For this review, take the finished solid that the model builds, in its own axes (mm). Round coordinates to 2 decimals unless told otherwise and drop trailing zeros. Loops run counter-clockwise (first coordinate to the right, second up) from the corner with the lowest first, then second, coordinate; pieces in that order, holes last.
1. Consider section C-C on x = 186. State the section outline as (y, z) points.
2. To check wall thickness, follow line 1 along Y through (x, z) = (236, -27); line 2 along Y through (x, z) = (59.5, -41); line 3 along Z through (x, y) = (119.5, -5). State the ranges of each line that lie inside material, in increasing order.
3. Clearance check with flat-ended pins moving along their axes: pin 1 Ø10 at (x, z) = (93.5, -4) entering from +Y; pin 2 Ø1.5 at (x, z) = (66.5, -39.5) entering from -Y; pin 3 Ø8 at (x, y) = (265, -23.5) entering from -Z. State where each tip first meets the part, or that it passes through.
4. Consider section B-B on z = -31. State the section outline as (x, y) points, then the cut area to 3 significant figures.
Autodesk Inventor part; units mm, degrees
ref_plane "YZ Plane" through (0, 0, 0) normal (1, 0, 0) x (0, 1, 0)
ref_plane "XZ Plane" through (0, 0, 0) normal (0, 1, 0) x (-1, 0, 0)
ref_plane "XY Plane" through (0, 0, 0) normal (0, 0, 1) x (1, 0, 0)
sketch "草圖3" plane through (0, 0, 0) normal (0, 1, 0) x (-1, 0, 0)
  line L0 (0, 50) -> (-450, 50)
  line L1 (-450, 50) -> (-450, -50)
  line L2 (-450, -50) -> (0, -50)
  line L3 (0, -50) -> (0, 50)
  point P0 (0, 0)
  point P1 (0, 0)
  dimension "d17" = 100
  dimension "d18" = 450
extrude "擠出3" add sketch "草圖3" along normal mid plane 100
chamfer "倒角4" distance 50 distance2 70 1 edges at (0, 0, 50) measured on face at (0, -16.6667, -16.6667)
chamfer "倒角5" distance 70 distance2 50 1 edges at (0, -50, -25) measured on face at (173.3333, -50, -16.6667)
chamfer "倒角6" distance 70 distance2 50 1 edges at (0, 25, -50) measured on face at (173.3333, 16.6667, -50)
chamfer "倒角8" distance 50 distance2 380 1 edges at (450, 0, -50) measured on face at (450, 16.6667, -16.6667)
chamfer "倒角9" distance 380 distance2 50 1 edges at (450, 50, 25) measured on face at (196.6667, 50, 0)
chamfer "倒角10" distance 50 distance2 380 1 edges at (450, -25, 50) measured on face at (450, -33.3333, 33.3333)
sketch "草圖4" plane through (0, 0, 0) normal (0, 0, 1) x (1, 0, 0)
  line L0 (450, -50) -> (70, -50)
  line L1 (450, 0) -> (70, 50)
  line L2 (70, -50) -> (450, 0)
  line L3 (450, 0) -> (450, -50)
  line L4 (450, 0) -> (450, -50)
  line L5 (450, -50) -> (70, -50)
  point P0 (0, 0)
  point P1 (70, 50)
  point P2 (170, -50)
  point P3 (170, 50)
extrude "擠出4" cut sketch "草圖4" along normal mid plane 100
sketch "草圖5" plane through (0, 0, 0) normal (0, 0, 1) x (1, 0, 0)
  line L0 (70, -50) -> (0, 0)
  line L1 (0, 50) -> (0, 0)
  line L2 (0, 0) -> (0, 50)
  line L3 (70, 50) -> (70, -50)
  line L4 (0, 50) -> (70, 50)
  line L5 (70, 50) -> (0, 0)
extrude "擠出5" cut sketch "草圖5" along normal mid plane 100 contours L1 L4 L5
sketch "草圖6" plane through (0, 0, 0) normal (1, 0, 0) x (0, 1, 0)
  circle A0 centre (0, 0) radius 25
  line L0 (0, 25) -> (0, -25)
  point P0 (0, 0)
  dimension "d46" = 50
revolve "迴轉1" add sketch "草圖6" angle 360 about axis through (0, 0, 25) along (0, 0, -1) picked at (-8.8525, -4.4917) contours L0 A0
sketch "草圖7" plane through (0, 0, 0) normal (0, 1, 0) x (-1, 0, 0)
  line L0 (-450, 0) -> (-70, -50)
  circle A0 centre (-450, 0) radius 15
  line L1 (-450, 15) -> (-450, -15)
  point P0 (0, 0)
  dimension "d48" = 30
revolve "迴轉2" add sketch "草圖7" angle 360 about axis through (450, 0, 15) along (0, 0, -1) contours L1 A0
properties part number "Bone"
Resolved:
1. outline: (-34.74, -34.74) - (34.74, -34.74) - (34.74, 34.74) - (-34.74, 34.74) - close
2. line 1: y = -28.16 to 28.16
2. line 2: y = -42.5 to 42.5
2. line 3: z = -43.49 to 43.49
3. pin 1: stops at y = 47.57
3. pin 2: stops at y = -48.04
3. pin 3: stops at z = -24.87
4. outline: (43.4, -31) - (70, -50) - (214.4, -31) - (214.4, 31) - (70, 50) - (43.4, 31) - close
4. area: 13,900 mm2
